Design review of the part built by this model. Coordinates are the model's own, in mm. A direction names the side the tool comes from. Give positions to 0.01 mm unless a question says otherwise; leave off trailing zeros. Loops run counter-clockwise (first coordinate to the right, second up) from the corner with the lowest first, then second, coordinate; pieces in that order, holes last. Notation, with made-up numbers: M 80,51.25 L 137,51.25 A26 cw 137,85.25 Z; hole C 37.25,4 d4. An arc over 180 degrees is marked long. Use a Markdown table: item, result. Add a question column.
(1) For probe 1 along Z at (x, y) = (0, -1.5); probe 2 along X at (y, z) = (-4.5, 0); probe 3 along Z at (x, y) = (0, -5.45), list the stretches that pass through material, from the lowest coordinate up.
(2) Add section D-D, the plane x = -26. Give the boundary of the cut face in (y, z).
(3) Draft analysis for pull direction Z (two halves, no side actions). For faces 3 (the face through (-19.45, -5.99, 19.8)), 4 (the face through (25, -5, 13)), 5 (the face through (0, -3, 21)), state which applies: pulls with the +Z half, pulls with the -Z half, needs draft (parallel to the pull), parting line crosses it, or undercut.
(4) Add section C-C, the plane x = 16. Give the boundary of the cut face in (y, z), then the cut area to 3 significant figures.
(5) For faces 1 (the face through (19.8, -5.99, 19.45)), 2 (the face through (-14.06, -3.451, 12.884)), list the 3-axis set-ups (+Z, -Z, +X, -X, +Y, -Y) from which the entire face can be reached by the end or side of a thin tool; tool diameter is ignored.
(6) Insertion check: pin 1 Ø1.5 at (x, y) = (22, -1) entering from -Z; pin 2 Ø9.5 at (x, z) = (-35, 0) entering from +Y; pin 3 Ø4 at (x, z) = (0, 23.5) entering from +Y; pin 4 Ø4 at (y, z) = (-6, -16.5) entering from -X. Each pin has a flat end and moves straight along its axis. Give the tip position at first contact, or say it passes through.
(7) Add section B-B, the plane y = -3. State how many separate pieces and enclosed holes the cut face has, then the cut area to 3 significant figures.
(8) Add section A-A, the plane z = 0. Give the boundary of the cut face in (x, y).
```python
from build123d import *

# Parameters (mm, degrees)
SKETCH1_R           = 27.5
BOSS_EXTRUDE1_DEPTH = 5
SKETCH2_R           = 42.5
BOSS_EXTRUDE2_DEPTH = 2
SKETCH3_R           = 3
CUT_EXTRUDE1_DEPTH  = 2
SKETCH4_R           = 11.6
SKETCH4_R_2         = 2.5
CUT_EXTRUDE2_DEPTH  = 8
CUT_EXTRUDE3_DEPTH  = 8
FILLET1_R           = 10


with BuildPart() as part:
    # Sketch1 → Boss-Extrude1 (new body)
    with BuildSketch(Plane(origin=(0, 0, 0), x_dir=(1, 0, 0), z_dir=(0, 1, 0))):
        Circle(SKETCH1_R)
    extrude(amount=-BOSS_EXTRUDE1_DEPTH)

    # Sketch2 → Boss-Extrude2 (add)
    with BuildSketch(Plane.XZ.offset(5)):
        Circle(SKETCH2_R)
    extrude(amount=BOSS_EXTRUDE2_DEPTH)

    # Sketch3 → Cut-Extrude1 (cut)
    with BuildSketch(Plane(origin=(0, -5, 0), x_dir=(1, 0, 0), z_dir=(0, 1, 0))):
        with BuildLine():
            ThreePointArc((-41.306779105, 10), (-19.624107624, 19.624107624), (-10, 41.306779105))
            ThreePointArc((-10, 41.306779105), (-30.0520382, 30.0520382), (-41.306779105, 10))
        make_face()
        with Locations((0, 35)):
            Circle(SKETCH3_R)
        with BuildLine():
            ThreePointArc((41.306779105, 10), (30.0520382, 30.0520382), (10, 41.306779105))
            ThreePointArc((10, 41.306779105), (19.624107624, 19.624107624), (41.306779105, 10))
        make_face()
        with Locations((35, 0)):
            Circle(SKETCH3_R)
        with Locations((0, -35)):
            Circle(SKETCH3_R)
        with BuildLine():
            ThreePointArc((41.306779105, -10), (19.624107624, -19.624107624), (10, -41.306779105))
            ThreePointArc((10, -41.306779105), (30.0520382, -30.0520382), (41.306779105, -10))
        make_face()
        with BuildLine():
            ThreePointArc((-10, -41.306779105), (-19.624107624, -19.624107624), (-41.306779105, -10))
            ThreePointArc((-41.306779105, -10), (-30.0520382, -30.0520382), (-10, -41.306779105))
        make_face()
        with Locations((-35, 0)):
            Circle(SKETCH3_R)
    extrude(amount=-CUT_EXTRUDE1_DEPTH, mode=Mode.SUBTRACT)

    # Sketch4 → Cut-Extrude2 (cut, through all)
    with BuildSketch(Plane(origin=(0, 0, 0), x_dir=(1, 0, 0), z_dir=(0, 1, 0))):
        Circle(SKETCH4_R)
        with Locations((0, 23.5)):
            Circle(SKETCH4_R_2)
        with Locations((20.351596989, 11.75)):
            Circle(SKETCH4_R_2)
        with Locations((20.351596989, -11.75)):
            Circle(SKETCH4_R_2)
        with Locations((0, -23.5)):
            Circle(SKETCH4_R_2)
        with Locations((-20.351596989, -11.75)):
            Circle(SKETCH4_R_2)
        with Locations((-20.351596989, 11.75)):
            Circle(SKETCH4_R_2)
    extrude(amount=-CUT_EXTRUDE2_DEPTH, mode=Mode.SUBTRACT)

    # Sketch5 → Cut-Extrude3 (cut, through all)
    with BuildSketch(Plane(origin=(0, 0, 0), x_dir=(1, 0, 0), z_dir=(0, 1, 0))):
        with BuildLine():
            Line((-17.694656083, 16.214164983), (-10.321882715, 9.458262907))
            ThreePointArc((-10.321882715, 9.458262907), (-7, 12.124355653), (-3.030154595, 13.6681441))
            Line((-3.030154595, 13.6681441), (-5.194550735, 23.431104171))
            ThreePointArc((-5.194550735, 23.431104171), (-12, 20.784609691), (-17.694656083, 16.214164983))
        make_face()
        with BuildLine():
            Line((17.694656083, 16.214164983), (10.321882715, 9.458262907))
            ThreePointArc((10.321882715, 9.458262907), (7, 12.124355653), (3.030154595, 13.6681441))
            Line((3.030154595, 13.6681441), (5.194550735, 23.431104171))
            ThreePointArc((5.194550735, 23.431104171), (12, 20.784609691), (17.694656083, 16.214164983))
        make_face()
        with BuildLine():
            Line((22.889206818, -7.216939188), (13.35203731, -4.209881193))
            ThreePointArc((13.35203731, -4.209881193), (14, 0), (13.35203731, 4.209881193))
            Line((13.35203731, 4.209881193), (22.889206818, 7.216939188))
            ThreePointArc((22.889206818, 7.216939188), (24, 0), (22.889206818, -7.216939188))
        make_face()
        with BuildLine():
            Line((5.194550735, -23.431104171), (3.030154595, -13.6681441))
            ThreePointArc((3.030154595, -13.6681441), (7, -12.124355653), (10.321882715, -9.458262907))
            Line((10.321882715, -9.458262907), (17.694656083, -16.214164983))
            ThreePointArc((17.694656083, -16.214164983), (12, -20.784609691), (5.194550735, -23.431104171))
        make_face()
        with BuildLine():
            Line((-17.694656083, -16.214164983), (-10.321882715, -9.458262907))
            ThreePointArc((-10.321882715, -9.458262907), (-7, -12.124355653), (-3.030154595, -13.6681441))
            Line((-3.030154595, -13.6681441), (-5.194550735, -23.431104171))
            ThreePointArc((-5.194550735, -23.431104171), (-12, -20.784609691), (-17.694656083, -16.214164983))
        make_face()
        with BuildLine():
            Line((-22.889206818, 7.216939188), (-13.35203731, 4.209881193))
            ThreePointArc((-13.35203731, 4.209881193), (-14, 0), (-13.35203731, -4.209881193))
            Line((-13.35203731, -4.209881193), (-22.889206818, -7.216939188))
            ThreePointArc((-22.889206818, -7.216939188), (-24, 0), (-22.889206818, 7.216939188))
        make_face()
    extrude(amount=-CUT_EXTRUDE3_DEPTH, mode=Mode.SUBTRACT)

    # Fillet1
    fillet1_edges = [part.edges().sort_by_distance(p)[0] for p in [
        (41.306779105, -6, -10),
        (10, -6, -41.306779105),
        (10, -6, 41.306779105),
        (41.306779105, -6, 10),
        (-41.306779105, -6, 10),
        (-10, -6, 41.306779105),
        (-10, -6, -41.306779105),
        (-41.306779105, -6, -10),
    ]]
    fillet(fillet1_edges, radius=FILLET1_R)


solid = part.part
```
Established:
| question | item | result |
|---|---|---|
| 1 | probe 1 | -27.5 to -26, -21 to -11.6, 11.6 to 21, 26 to 27.5 |
| 1 | probe 2 | -27.5 to -24, -14 to -11.6, 11.6 to 14, 24 to 27.5 |
| 1 | probe 3 | -42.5 to -38, -32 to -26, -21 to -11.6, 11.6 to 21, 26 to 32, 38 to 42.5 |
| 2 | outline | M -7,-14.65 L -5,-14.65 L -5,-8.96 L 0,-8.96 L 0,8.96 L -5,8.96 L -5,14.65 L -7,14.65 Z |
| 3 | face 3 | pulls with the +Z half |
| 3 | face 4 | needs draft |
| 3 | face 5 | undercut |
| 4 | outline | M -7,-23.93 L -5,-23.93 L -5,-22.37 L 0,-22.37 L 0,-17.89 L -7,-17.89 Z; M -7,-14.66 L 0,-14.66 L 0,-5.04 L -7,-5.04 Z; M -7,5.04 L 0,5.04 L 0,14.66 L -7,14.66 Z; M -7,17.89 L 0,17.89 L 0,22.37 L -5,22.37 L -5,23.93 L -7,23.93 Z |
| 4 | area | 204 mm^2 |
| 5 | face 1 | +Z, +X, +Y, -Y |
| 5 | face 2 | +Y, -Y |
| 6 | pin 1 | z = -17.46 |
| 6 | pin 2 | y = -5 |
| 6 | pin 3 | through |
| 6 | pin 4 | x = -26.25 |
| 7 | separate pieces | 1 |
| 7 | enclosed holes | 13 |
| 7 | area | 1,140 mm^2 |
| 8 | outline | M -42.5,-7 L -38,-7 L -38,-5 L -42.5,-5 Z; M -32,-7 L -24,-7 L -24,0 L -27.5,0 L -27.5,-5 L -32,-5 Z; M -14,-7 L -11.6,-7 L -11.6,0 L -14,0 Z; M 11.6,-7 L 14,-7 L 14,0 L 11.6,0 Z; M 24,-7 L 32,-7 L 32,-5 L 27.5,-5 L 27.5,0 L 24,0 Z; M 38,-7 L 42.5,-7 L 42.5,-5 L 38,-5 Z |
